Part model, mm, in its own coordinate system. A direction names the side the tool comes from. Round coordinates to 2 decimals unless told otherwise and drop trailing zeros. Loops run counter-clockwise (first coordinate to the right, second up) from the corner with the lowest first, then second, coordinate; pieces in that order, holes last. Notation, with made-up numbers: M 57,10 L 79,10 A23 cw 79,45 Z; hole C -17,24 d7. An arc over 180 degrees is marked long. Answer as CSV lines item,"result". Start each with the question number.
Item 1: Band-saw the part on B-B (z = -8). Give the cut face in (x, y), and give its area (3 significant figures).
Item 2: Drop a flat-ended pin along its axis: pin 1 Ø3 at (x, z) = (-22.3, 19.1) entering from +Y. Give the stop position or say it passes through.
Item 3: Mould opens along Z. For faces 1 (the flat face through (96, -2, -1)), 2 (the flat face through (81, -2, -68)), 3 (the flat face through (1, -2, 73)) say: pulls with the +Z half, pulls with the -Z half, needs draft (parallel to the pull), parting line crosses it, or undercut.
Item 4: Band-saw the part on C-C (x = 45). Give the cut face in (y, z), and give its area (3 significant figures).
Item 5: Band-saw the part on D-D (y = -4.2). Count the separate pieces of the cut face and the enclosed holes in it, and give its area (3 significant figures).
Item 6: Which spindle directions (+Z, -Z, +X, -X, +Y, -Y) get a long thin tool onto all of the face, cutting with end or side? Do faces 4 (the flat face through (72, -2, -70)), 5 (the flat face through (-1, -5, 1)). Say none if no direction does.
Item 7: Band-saw the part on A-A (x = -12.5). Give the cut face in (y, z), and give its area (3 significant figures).
Item 8: Wall check: line 1 (Z direction, x = 5, y = -0.95); line 2 (Z direction, x = -17.9, y = -3.7); line 3 (Z direction, x = -79.5, y = -1.35). Give the ranges that are in metal, low to high.
```python
from build123d import *

# Parameters (mm, degrees)
F0_W     = 18
F0_H     = 5
F0_W_2   = 5
F0_H_2   = 18
F0_R     = 1.75
F0_R_2   = 29.5
F0_W_3   = 30
F0_H_3   = 22
F1_DEPTH = 5


with BuildPart() as f1:
    # F0 (on Front) → F1 (new body)
    with BuildSketch(Plane.XZ):
        with BuildLine():
            Line((93, 73), (-93, 73))
            ThreePointArc((-93, 73), (-95.12132, 72.12132), (-96, 70))
            Line((-96, 70), (-96, -70))
            ThreePointArc((-96, -70), (-95.12132, -72.12132), (-93, -73))
            Line((-93, -73), (93, -73))
            ThreePointArc((93, -73), (95.12132, -72.12132), (96, -70))
            Line((96, -70), (96, 70))
            ThreePointArc((96, 70), (95.12132, 72.12132), (93, 73))
        make_face()
        with Locations((-72, -67.5)):
            Rectangle(F0_W, F0_H, mode=Mode.SUBTRACT)
        with Locations((-90.5, -49)):
            Rectangle(F0_W_2, F0_H_2, mode=Mode.SUBTRACT)
        with Locations((-67.7, -35.1)):
            Circle(F0_R, mode=Mode.SUBTRACT)
        with Locations((-17.9, -30.7)):
            Circle(F0_R, mode=Mode.SUBTRACT)
        with Locations((-45, -8)):
            Circle(F0_R_2, mode=Mode.SUBTRACT)
        with Locations((72, -67.5)):
            Rectangle(F0_W, F0_H, mode=Mode.SUBTRACT)
        with Locations((90.5, -49)):
            Rectangle(F0_W_2, F0_H_2, mode=Mode.SUBTRACT)
        with Locations((22.3, -35.1)):
            Circle(F0_R, mode=Mode.SUBTRACT)
        with Locations((45, -8)):
            Circle(F0_R_2, mode=Mode.SUBTRACT)
        with Locations((72.1, -30.7)):
            Circle(F0_R, mode=Mode.SUBTRACT)
        with Locations((-72.1, 14.7)):
            Circle(F0_R, mode=Mode.SUBTRACT)
        with Locations((-22.3, 19.1)):
            Circle(F0_R, mode=Mode.SUBTRACT)
        with Locations((-90.5, 49)):
            Rectangle(F0_W_2, F0_H_2, mode=Mode.SUBTRACT)
        with Locations((-72, 67.5)):
            Rectangle(F0_W, F0_H, mode=Mode.SUBTRACT)
        with Locations((17.9, 14.7)):
            Circle(F0_R, mode=Mode.SUBTRACT)
        with Locations((67.7, 19.1)):
            Circle(F0_R, mode=Mode.SUBTRACT)
        with Locations((0, 52)):
            Rectangle(F0_W_3, F0_H_3, mode=Mode.SUBTRACT)
        with Locations((90.5, 49)):
            Rectangle(F0_W_2, F0_H_2, mode=Mode.SUBTRACT)
        with Locations((72, 67.5)):
            Rectangle(F0_W, F0_H, mode=Mode.SUBTRACT)
        with Locations((-72, 67.5)):
            Rectangle(F0_W, F0_H)
        with Locations((72, 67.5)):
            Rectangle(F0_W, F0_H)
    extrude(amount=F1_DEPTH)


solid = f1.part
```
Answer block:
1,outline,"M -96,-5 L -74.5,-5 L -74.5,0 L -96,0 Z; M -15.5,-5 L 15.5,-5 L 15.5,0 L -15.5,0 Z; M 74.5,-5 L 96,-5 L 96,0 L 74.5,0 Z"
1,area,"370 mm^2"
2,pin 1,"passes through"
3,face 1,"needs draft"
3,face 2,"undercut"
3,face 3,"pulls with the +Z half"
4,outline,"M -5,-73 L 0,-73 L 0,-37.5 L -5,-37.5 Z; M -5,21.5 L 0,21.5 L 0,73 L -5,73 Z"
4,area,"435 mm^2"
5,separate pieces,"1"
5,enclosed holes,"17"
5,area,"21,300 mm^2"
6,face 4,"+Y, -Y"
6,face 5,"+Z, -Z, +X, -X, -Y"
7,outline,"M -5,-73 L 0,-73 L 0,41 L -5,41 Z; M -5,63 L 0,63 L 0,73 L -5,73 Z"
7,area,"620 mm^2"
8,line 1,"z = -73 to 41, 63 to 73"
8,line 2,"z = -73 to -32.45, -28.95 to -19.66, 3.66 to 73"
8,line 3,"z = -73 to -70, -65 to 73"
